Could you check a few things on this model? Use its own coordinates, in mm. Face numbers are marked on the shaded views. A direction names the side the tool comes from. Coordinates: 2 decimals unless noted, no trailing zeros. Loops run counter-clockwise (first coordinate to the right, second up) from the corner with the lowest first, then second, coordinate; pieces in that order, holes last. Notation, with made-up numbers: M 9,-23.5 L 19,-23.5 A14 ccw 19,-4.5 Z; hole C -32.75,88.5 d4. An arc over 180 degrees is marked long. Return JSON: item names as keys, results as strings. Group by question number.
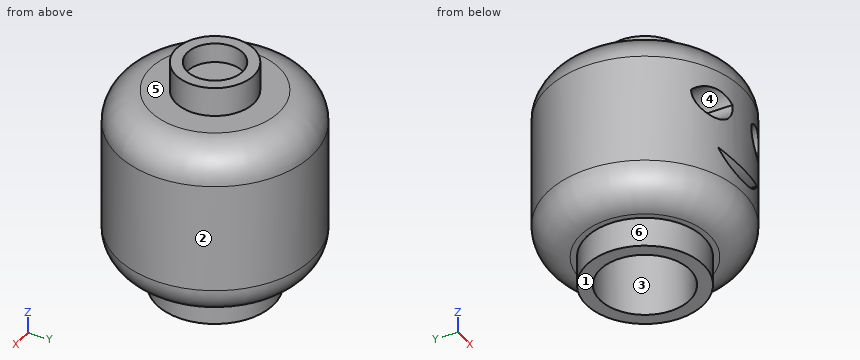
from build123d import *

# Parameters (mm, degrees)
F0_R      = 3
F1_DEPTH  = 12
F2_R      = 3.203206237
F2_R_2    = 1.9962564084
F3_DEPTH  = 1.5
F4_R      = 5
F5_DEPTH  = 9
F6_R      = 1.7
F7_R      = 1.4223649875
F8_DEPTH  = 1
F9_R      = 2.3001696125
F10_DEPTH = 5
F12_DEPTH = 25
F13_DEPTH = 3


with BuildPart() as f1:
    # F0 (on Top) → F1 (new body)
    with BuildSketch(Plane.XY):
        Circle(F0_R)
    extrude(amount=-F1_DEPTH)

    # F2 (on face) → F3 (cut)
    with BuildSketch(Plane.XY):
        Circle(F2_R)
        Circle(F2_R_2, mode=Mode.SUBTRACT)
    extrude(amount=-F3_DEPTH, mode=Mode.SUBTRACT)

    # F4 (on face) → F5 (join)
    with BuildSketch(Plane.XY.offset(-1.5)):
        Circle(F4_R)
    extrude(amount=-F5_DEPTH)

    # F6
    f6_edges = [f1.edges().sort_by_distance(p)[0] for p in [
        (5, 0, -6),
        (-5, 0, -1.5),
        (-5, 0, -10.5),
    ]]
    fillet(f6_edges, radius=F6_R)

    # F7 (on face) → F8 (cut)
    with BuildSketch(Plane.XY):
        Circle(F7_R)
    extrude(amount=-F8_DEPTH, mode=Mode.SUBTRACT)

    # F9 (on face) → F10 (cut)
    with BuildSketch(Plane(origin=(0, 0, -12), x_dir=(1, 0, 0), z_dir=(0, 0, -1))):
        Circle(F9_R)
    extrude(amount=-F10_DEPTH, mode=Mode.SUBTRACT)

    # F11 (on Front) → F12 (cut)
    with BuildSketch(Plane.XZ):
        with BuildLine():
            ThreePointArc((1.7097895663, -7.2849687191), (-0.003580854, -7.5244880061), (-1.715676859, -7.2760228068))
            ThreePointArc((-1.715676859, -7.2760228068), (-0.0053546607, -8.2036937796), (1.7097895663, -7.2849687191))
        make_face()
        with BuildLine():
            ThreePointArc((-2.9485186096, -4.6888017096), (-1.8248803235, -5.7631106344), (-0.84451411, -4.5566344634))
            ThreePointArc((-0.84451411, -4.5566344634), (-1.924158161, -4.1826811203), (-2.9485186096, -4.6888017096))
        make_face()
        with BuildLine():
            ThreePointArc((0.8465747233, -4.5566344634), (1.7231712571, -5.7150981177), (2.7513615138, -4.6888017096))
            ThreePointArc((2.7513615138, -4.6888017096), (1.826312953, -4.2286258966), (0.8465747233, -4.5566344634))
        make_face()
    extrude(amount=F12_DEPTH, mode=Mode.SUBTRACT)

    # F13 (add): faces of the model
    f13_faces = [f1.faces().sort_by_distance(p)[0] for p in [
        (-1.8763016609, 0, -4.9445210943),
        (1.7765781537, 0, -4.9454009795),
    ]]
    extrude(f13_faces, amount=F13_DEPTH)


solid = f1.part
(1) For the marked faces 4, 5 and 6, which set-ups out of +Z, -Z, +X, -X, +Y, -Y let a thin tool reach every point of the face, with its end or its side?
(2) Imagine slicing it at C-C, the plane z = -8.5. Write out the boundary of the cut face in (x, y).
(3) Imagine slicing it at A-A, the plane y = 0. Write out the boundary of the cut face in (x, z).
(4) Imagine slicing it at B-B, the plane x = 0. Write out the boundary of the cut face in (y, z), then the cut area to 3 significant figures.
(5) If I drill on L1, parallel to Y at x = 0, z = -0.3; L2, parallel to Z at x = 0, y = -2.25; L3, parallel to Z at x = -2.5, y = -0.75, over which ranges is the centre line in solid material (lowest first)? Write a range as [from, to].
(6) We'd pull the mould along X, two halves only. Please class the marked faces 1, 2 and 3: +X half, -X half, draft (parallel to the pull), parting line (faces both ways), or undercut.
(7) Will these pins go through, and if not, where does the flat tip stop? P1, Ø5, axis at x = 2.5, z = -5, coming from the +Y side; P2, Ø3, axis at x = 3, z = -1.5, coming from the -Y side; P3, Ø3, axis at x = 0, y = 0, coming from the -Z side; P4, Ø0.5, axis at x = -2, z = -5, coming from the -Y side.
Checks:
{
 "1": {"face 4": "-Y", "face 5": "+Z", "face 6": "-Z"},
 "2": {"outline": "C 0,0 d10; hole C 0,0 d4.6"},
 "3": {"outline": "M -5,-8.8 A1.7 ccw -3.3,-10.5 L -3,-10.5 L -3,-12 L -2.3,-12 L -2.3,-7 L 2.3,-7 L 2.3,-12 L 3,-12 L 3,-10.5 L 3.3,-10.5 A1.7 ccw 5,-8.8 L 5,-3.2 A1.7 ccw 3.3,-1.5 L 2,-1.5 L 2,0 L 1.42,0 L 1.42,-1 L -1.42,-1 L -1.42,0 L -2,0 L -2,-1.5 L -3.3,-1.5 A1.7 ccw -5,-3.2 Z"},
 "4": {"outline": "M -5,-8.8 A1.7 ccw -3.3,-10.5 L -3,-10.5 L -3,-12 L -2.3,-12 L -2.3,-8.2 L -5,-8.2 Z; M -5,-7.52 L -2.3,-7.52 L -2.3,-7 L 2.3,-7 L 2.3,-12 L 3,-12 L 3,-10.5 L 3.3,-10.5 A1.7 ccw 5,-8.8 L 5,-3.2 A1.7 ccw 3.3,-1.5 L 2,-1.5 L 2,0 L 1.42,0 L 1.42,-1 L -1.42,-1 L -1.42,0 L -2,0 L -2,-1.5 L -3.3,-1.5 A1.7 ccw -5,-3.2 Z", "area": "74.8 mm²"},
 "5": {"L1": "[-2, -1.42], [1.42, 2]", "L2": "[-7, -1.5]", "L3": "[-12, -1.5]"},
 "6": {"face 1": "draft", "face 2": "parting line", "face 3": "undercut"},
 "7": {"P1": "y = 5", "P2": "y = -4.47", "P3": "z = -7", "P4": "y = -3"}
}
